```python
from build123d import *

# Parameters (mm, degrees)
SKETCH1_R                = 2.1717
BOSS_EXTRUDE2_DEPTH      = 2.54
BOSS_EXTRUDE3_DEPTH      = 25.4
BOSS_EXTRUDE3_DEPTH_BACK = 2.54
SKETCH2_W                = 10.16
SKETCH2_H                = 7.62
SKETCH3_W                = 5.08
SKETCH3_H                = 2.54
BOSS_EXTRUDE7_DEPTH      = 12.7
BOSS_EXTRUDE8_DEPTH      = 5.08


with BuildPart() as part:
    # Sketch1 → Boss-Extrude2 (new body)
    with BuildSketch(Plane.XY):
        Polygon((10.102114399, -10.102114399), (46.910827705, -10.102114399), (51.562, -5.08), (61.722, -5.08), (61.722, 5.08), (56.642, 5.08), (51.562, 5.08), (46.252389936, -5.08), (12.145313508, -5.08), (5.08, 5.08), (0, 5.08), (-5.08, 5.08), (-5.08, -5.08), (5.08, -5.08), align=None)
        with Locations((56.642, 0)):
            Circle(SKETCH1_R, mode=Mode.SUBTRACT)
        Circle(SKETCH1_R, mode=Mode.SUBTRACT)
    extrude(amount=BOSS_EXTRUDE2_DEPTH)

    # Sketch2 → Boss-Extrude3 (add, two sides: drawn at the far end of the back side and taken through both)
    with BuildSketch(Plane.XY.offset(2.54).offset(-BOSS_EXTRUDE3_DEPTH_BACK)):
        with Locations((0, -8.89)):
            Rectangle(SKETCH2_W, SKETCH2_H)
    extrude(amount=BOSS_EXTRUDE3_DEPTH + BOSS_EXTRUDE3_DEPTH_BACK)

    # Sketch3 → Boss-Extrude7 (add)
    with BuildSketch(Plane.XY.offset(2.54)):
        with Locations((32.258, -6.35)):
            Rectangle(SKETCH3_W, SKETCH3_H)
    extrude(amount=BOSS_EXTRUDE7_DEPTH)

    # Sketch5 → Boss-Extrude8 (add)
    with BuildSketch(Plane(origin=(34.798, 0, 0), x_dir=(0, 0, -1), z_dir=(1, 0, 0))):
        Polygon((-15.24, -7.62), (-15.24, -12.7), (-13.97, -12.7), (-11.834830977, -12.7), (-11.938, -8.763360945), (-13.693199114, -8.763360945), (-13.693199114, -9.646415213), (-12.841122396, -9.646415213), (-12.841122396, -11.658511366), (-13.97, -12.215842923), (-13.97, -9.646415213), (-13.97, -7.62), align=None)
    extrude(amount=-BOSS_EXTRUDE8_DEPTH)


solid = part.part
```
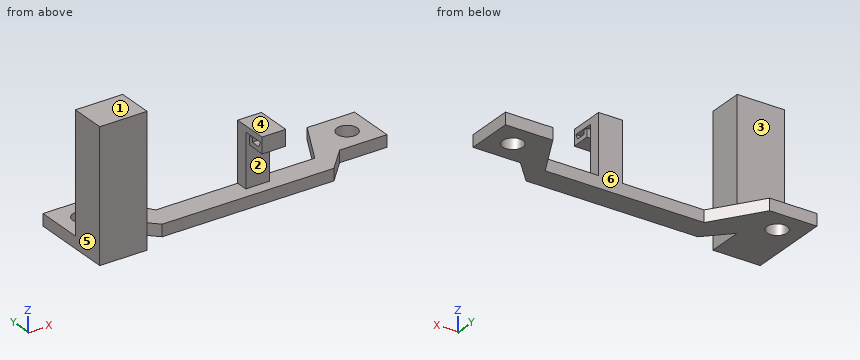
Input: part model. Units: mm. Frame: model coordinates. Face numbers are marked on the shaded views. A direction names the side the tool comes from. Give positions to 0.01 mm unless a question says otherwise; leave off trailing zeros. Order: outer loops, then holes, each group sorted by start corner. A loop starts at its lowest first (then second) coordinate and runs counter-clockwise, first axis right, second up. Notation, with made-up numbers: M -1,56.25 L 20,56.25 A14 ccw 20,63.25 Z; hole C 19.5,26 d5. An arc over 180 degrees is marked long. Return JSON: item names as keys, results as strings.
Item 1: First-contact query: P1, Ø1, axis at x = 32, y = -11, coming from the +Z side; P2, Ø7, axis at x = 56.642, y = 0, coming from the -Z side; P3, Ø1.5, axis at x = 33.5, z = 7.5, coming from the -Y side; P4, Ø0.8, axis at x = 56.5, z = 1, coming from the -Y side. Flat tips, straight axial feed; report the tip coordinate or a pass-through.
Solutions:
{"P1": "z = 15.24", "P2": "z = 0", "P3": "y = -7.62", "P4": "y = -5.08"}
Item 2: Access query for the marked faces 1, 2 and 3. Directions: +Z, -Z, +X, -X, +Y, -Y. A direction counts if a zero-diameter tool reaches every point of the face in a straight line with its end or side. Return the directions, or none.
Solutions:
{"face 1": "+Z, +X, -X, +Y, -Y", "face 2": "+X", "face 3": "+Z, +X, -X, +Y"}
Item 3: Cut plane A-A (x = 0). Return loops of the section in (y, z).
Solutions:
{"outline": "M -12.7,0 L -2.17,0 L -2.17,2.54 L -5.08,2.54 L -5.08,27.94 L -12.7,27.94 Z; M 2.17,0 L 5.08,0 L 5.08,2.54 L 2.17,2.54 Z"}
Item 4: Cut plane C-C (y = -6.5). Return loops of the section in (x, z), then the cut area to 3 significant figures.
Solutions:
{"outline": "M -5.08,0 L 5.08,0 L 5.08,27.94 L -5.08,27.94 Z; M 6.5,0 L 50.25,0 L 50.25,2.54 L 34.8,2.54 L 34.8,15.24 L 29.72,15.24 L 29.72,2.54 L 6.5,2.54 Z", "area": "460 mm^2"}
Item 5: Cut plane D-D (x = 32). Return loops of the section in (y, z).
Solutions:
{"outline": "M -12.7,11.83 L -8.76,11.94 L -8.76,13.69 L -9.65,13.69 L -9.65,12.84 L -11.66,12.84 L -12.22,13.97 L -7.62,13.97 L -7.62,2.54 L -10.1,2.54 L -10.1,0 L -5.08,0 L -5.08,15.24 L -12.7,15.24 Z"}
Item 6: Ray query, probe 1 along Y at (x, z) = (0, 1.9); probe 2 along X at (y, z) = (-8.25, 14.5); probe 3 along Y at (x, z) = (1.5, 1.5). Return the intervals inside material, ascending.
Solutions:
{"probe 1": "-12.7 to -2.17, 2.17 to 5.08", "probe 2": "-5.08 to 5.08, 29.72 to 34.8", "probe 3": "-12.7 to -1.57, 1.57 to 5.08"}
Item 7: Cut plane B-B (y = 0). Return loops of the section in (x, z), then the cut area to 3 significant figures.
Solutions:
{"outline": "M -5.08,0 L -2.17,0 L -2.17,2.54 L -5.08,2.54 Z; M 2.17,0 L 8.61,0 L 8.61,2.54 L 2.17,2.54 Z; M 48.91,0 L 54.47,0 L 54.47,2.54 L 48.91,2.54 Z; M 58.81,0 L 61.72,0 L 61.72,2.54 L 58.81,2.54 Z", "area": "45.3 mm^2"}
Item 8: Pull-direction query (X, two-part tool) for the marked faces 4, 5 and 6; classes: +X half, -X half, draft (parallel to the pull), parting line (faces both ways), or undercut.
Solutions:
{"face 4": "draft", "face 5": "-X half", "face 6": "undercut"}
